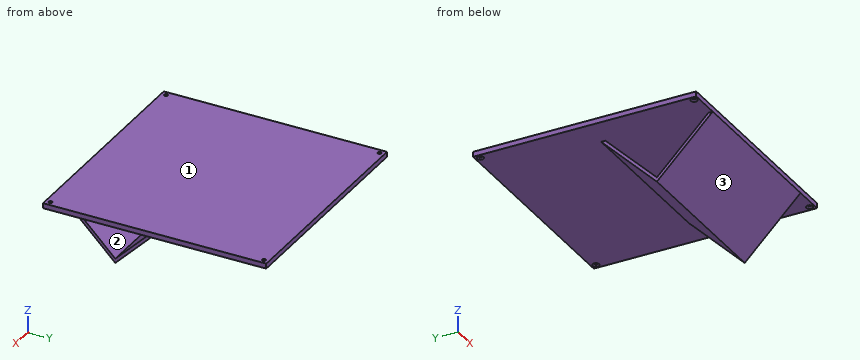
from build123d import *

# Parameters (mm, degrees)
SKICA1_W                                          = 220
SKICA1_H                                          = 220
P_IDAT_VYSUNUT_M1_DEPTH                           = 5
KU_ELOV_ZAHLOUBEN_PRO_M3_ROUBU_SE_Z_P_D           = 3.4
KU_ELOV_ZAHLOUBEN_PRO_M3_ROUBU_SE_Z_P_CSINK_D     = 6.3
KU_ELOV_ZAHLOUBEN_PRO_M3_ROUBU_SE_Z_P_CSINK_ANGLE = 90
ZRCADLIT1_AT_THE_SECOND_PLANE_COPY_1_D            = 3.4
ZRCADLIT1_AT_THE_SECOND_PLANE_COPY_1_CSINK_D      = 6.3
ZRCADLIT1_AT_THE_SECOND_PLANE_COPY_1_CSINK_ANGLE  = 90
SKICA11_W                                         = 160
SKICA11_H                                         = 77.7817
P_IDAT_VYSUNUT_M2_DEPTH                           = 3
SKICA17_W                                         = 160
SKICA17_H                                         = 77.781745931
P_IDAT_VYSUNUT_M3_DEPTH                           = 3


with BuildPart() as part:
    # Skica1 → Přidat vysunutím1 (new body)
    with BuildSketch(Plane.XY):
        Rectangle(SKICA1_W, SKICA1_H)
    extrude(amount=P_IDAT_VYSUNUT_M1_DEPTH)

    # Kuželové zahloubení pro M3 šroubu se zápustnou hlavou plochou1 (through all)
    with Locations(Plane(origin=(0, 0, 0), x_dir=(-1, 0, 0), z_dir=(0, 0, -1))):
        with Locations((-105.25, -105.25)):
            ku_elov_zahlouben_pro_m3_roubu_se_z_p = CounterSinkHole(KU_ELOV_ZAHLOUBEN_PRO_M3_ROUBU_SE_Z_P_D / 2, KU_ELOV_ZAHLOUBEN_PRO_M3_ROUBU_SE_Z_P_CSINK_D / 2, counter_sink_angle=KU_ELOV_ZAHLOUBEN_PRO_M3_ROUBU_SE_Z_P_CSINK_ANGLE)

    # Zrcadlit1: Kuželové zahloubení pro M3 šroubu se zápustnou hlavou plochou1 across plane
    add(ku_elov_zahlouben_pro_m3_roubu_se_z_p.mirror(Plane.ZX), mode=Mode.SUBTRACT)

    # Zrcadlit1 at the second plane: Kuželové zahloubení pro M3 šroubu se zápustnou hlavou plochou1 across plane
    add(ku_elov_zahlouben_pro_m3_roubu_se_z_p.mirror(Plane(origin=(0, 0, 0), x_dir=(0, 0, 1), z_dir=(1, 0, 0))), mode=Mode.SUBTRACT)

    # Zrcadlit1 at the second plane copy 1 (through all)
    with Locations(Plane(origin=(0, 0, 0), x_dir=(1, 0, 0), z_dir=(0, 0, -1))):
        with Locations((-105.25, -105.25)):
            CounterSinkHole(ZRCADLIT1_AT_THE_SECOND_PLANE_COPY_1_D / 2, ZRCADLIT1_AT_THE_SECOND_PLANE_COPY_1_CSINK_D / 2, counter_sink_angle=ZRCADLIT1_AT_THE_SECOND_PLANE_COPY_1_CSINK_ANGLE)

    # Skica11 → Přidat vysunutím2 (add)
    with BuildSketch(Plane(origin=(0, 0, 0), x_dir=(-1, 0, 0), z_dir=(0, -0.7071067811865438, 0.7071067811865512))):
        with Locations((0, 38.89085)):
            Rectangle(SKICA11_W, SKICA11_H)
    extrude(amount=P_IDAT_VYSUNUT_M2_DEPTH)

    # Skica17 → Přidat vysunutím3 (add)
    with BuildSketch(Plane(origin=(0, -54.999967522, -54.999967522), x_dir=(1, 0, 0), z_dir=(0, -0.7071067811865513, -0.7071067811865438))):
        with Locations((0, 38.890872966)):
            Rectangle(SKICA17_W, SKICA17_H)
    extrude(amount=-P_IDAT_VYSUNUT_M3_DEPTH)


solid = part.part
Design review of the part built by this model. Coordinates are the model's own, in mm. Face numbers are marked on the shaded views. Round coordinates to 2 decimals unless told otherwise and drop trailing zeros. Write each loop counter-clockwise with the first axis right and the second up, starting at its lowest first coordinate (ties: lowest second). Pieces come first, ordered by that corner, then holes. Notation, with made-up numbers: M 6.25,63 L 33.25,63 A17 cw 33.25,94 Z; hole C 53,28 d5. An arc over 180 degrees is marked long. One line per item, written item: value. Start each with the question number.
1. Take a section at B-B on z = -33. State the section outline as (x, y) points.
2. Take a section at C-C on y = 75. State the section outline as (x, z) points, then the cut area to 3 significant figures.
3. Draft analysis for pull direction Z (two halves, no side actions). For the marked faces 1, 2 and 3, state which applies: pulls with the +Z half, pulls with the -Z half, needs draft (parallel to the pull), parting line crosses it, or undercut.
4. To check wall thickness, follow probe 1 along X at (y, z) = (105, 2); probe 2 along Y at (x, z) = (105.25, 4.2); probe 3 along Z at (x, y) = (-27, 10.5). State the ranges of each line that lie inside material, in increasing order. Write a range as from..to.
5. Clearance check with flat-ended pins moving along their axes: P1, Ø4.5, axis at x = -105.25, y = -105.25, coming from the -Z side; P2, Ø2.5, axis at x = -105.25, y = 105.25, coming from the +Z side; P3, Ø5, axis at x = 42, z = -4.5, coming from the -Y side; P4, Ø12, axis at x = 16, z = -47.5, coming from the +Y side. State where each tip first meets the part, or that it passes through.
Computed:
1. outline: M -80,-77 L 80,-77 L 80,-72.76 L -80,-72.76 Z; M -80,-37.24 L 80,-37.24 L 80,-33 L -80,-33 Z
2. outline: M -110,0 L 110,0 L 110,5 L -110,5 Z
2. area: 1,100 mm²
3. face 1: pulls with the +Z half
3. face 2: undercut
3. face 3: pulls with the -Z half
4. probe 1: x = -110..-106.93, -103.57..103.57, 106.93..110
4. probe 2: y = -110..-106.95, -103.55..103.55, 106.95..110
4. probe 3: z = 0..5
5. P1: stops at z = 0.9
5. P2: passes through
5. P3: stops at y = -108
5. P4: stops at y = -41.5
